from build123d import *

# Parameters (mm, degrees)
SKETCH1_R           = 47.5
BOSS_EXTRUDE1_DEPTH = 100
SKETCH2_R           = 47.5
BOSS_EXTRUDE2_DEPTH = 62.5
SKETCH3_R           = 27
CUT_EXTRUDE1_DEPTH  = 4
HOLE1_D             = 10
HOLE1_DEPTH         = 20
SKETCH6_R           = 30
CUT_EXTRUDE2_DEPTH  = 200


with BuildPart() as part:
    # Sketch1 → Boss-Extrude1 (new body, symmetric)
    with BuildSketch(Plane.XY):
        Circle(SKETCH1_R)
    extrude(amount=BOSS_EXTRUDE1_DEPTH, both=True)

    # Sketch2 → Boss-Extrude2 (add)
    with BuildSketch(Plane(origin=(0, 0, 0), x_dir=(1, 0, 0), z_dir=(0, 1, 0))):
        Circle(SKETCH2_R)
    extrude(amount=BOSS_EXTRUDE2_DEPTH)

    # Sketch3 → Cut-Extrude1 (cut)
    with BuildSketch(Plane(origin=(0, 62.5, 0), x_dir=(1, 0, 0), z_dir=(0, 1, 0))):
        Circle(SKETCH3_R)
    extrude(amount=-CUT_EXTRUDE1_DEPTH, mode=Mode.SUBTRACT)

    # Hole1
    with Locations(Plane(origin=(38, 62.5, 0), x_dir=(0, 0, 1), z_dir=(0, 1, 0))):
        with Locations((0, 0), (-38, -38), (0, -76), (38, -38)):
            Hole(HOLE1_D / 2, depth=HOLE1_DEPTH)

    # Sketch6 → Cut-Extrude2 (cut)
    with BuildSketch(Plane(origin=(0, 0, -100), x_dir=(-1, 0, 0), z_dir=(0, 0, -1))):
        Circle(SKETCH6_R)
    extrude(amount=-CUT_EXTRUDE2_DEPTH, mode=Mode.SUBTRACT)


solid = part.part
Geometry: final body of the model. Coordinates: model frame, mm. A direction names the side the tool comes from. Give positions to 0.01 mm unless a question says otherwise; leave off trailing zeros. Write each loop counter-clockwise with the first axis right and the second up, starting at its lowest first coordinate (ties: lowest second). Pieces come first, ordered by that corner, then holes. Notation, with made-up numbers: (89.5, 56) -> (124.5, 56) arc R32 cw to (124.5, 85) -> close; hole circle Ø3 at (64.5, 35.25). An arc over 180 degrees is marked (long way). Answer as a JSON object with one key per item and string values.
1. Contact query for flat-ended pins moving along their axis: pin 1 (3 mm diameter, centred on x = -0.5, z = -40.5, fed in from +Y); pin 2 (3 mm diameter, centred on x = 23.5, z = 67.5, fed in from +Y); pin 3 (12 mm diameter, centred on x = 24, y = 45.5, fed in from +Z); pin 4 (5 mm diameter, centred on x = -37, z = 11, fed in from -Y). Output: stop coordinate, or through.
Ans:
{"pin 1": "stops at y = 42.5", "pin 2": "stops at y = 42.1", "pin 3": "stops at z = 100", "pin 4": "stops at y = -32.65"}
2. Cut plane B-B on x = 0. Output: boundary loops of the cut face in (y, z), and give its area (3 significant figures).
Ans:
{"outline": "(-47.5, -100) -> (-30, -100) -> (-30, 100) -> (-47.5, 100) -> close; (30, -100) -> (47.5, -100) -> (47.5, -47.5) -> (62.5, -47.5) -> (62.5, -43) -> (42.5, -43) -> (42.5, -33) -> (62.5, -33) -> (62.5, -27) -> (58.5, -27) -> (58.5, 27) -> (62.5, 27) -> (62.5, 33) -> (42.5, 33) -> (42.5, 43) -> (62.5, 43) -> (62.5, 47.5) -> (47.5, 47.5) -> (47.5, 100) -> (30, 100) -> close", "area": "7,810 mm^2"}
3. Cut plane A-A on z = 0. Output: boundary loops of the cut face in (x, y).
Ans:
{"outline": "(-47.5, 0) arc R47.5 ccw to (47.5, 0) -> (47.5, 62.5) -> (43, 62.5) -> (43, 42.5) -> (33, 42.5) -> (33, 62.5) -> (27, 62.5) -> (27, 58.5) -> (-27, 58.5) -> (-27, 62.5) -> (-33, 62.5) -> (-33, 42.5) -> (-43, 42.5) -> (-43, 62.5) -> (-47.5, 62.5) -> close; hole circle Ø60 at (0, 0)"}
4. Cut plane D-D on x = 38. Output: boundary loops of the cut face in (y, z).
Ans:
{"outline": "(-28.5, -100) -> (28.5, -100) -> (28.5, -28.5) -> (62.5, -28.5) -> (62.5, -5) -> (42.5, -5) -> (42.5, 5) -> (62.5, 5) -> (62.5, 28.5) -> (28.5, 28.5) -> (28.5, 100) -> (-28.5, 100) -> close"}
5. Mould query, pull axis Y, two halves, no side actions, for faces 3 (the cylindrical face through (-34, 52, -3)), 4 (the flat face through (-38, 42.5, 0)), 5 (the cylindrical face through (-10.3, -46.37, 1.4)), 6 (the cylindrical face through (29.97, 1.32, -1.4)). Classes: pulls with the +Y half, pulls with the -Y half, needs draft (parallel to the pull), parting line crosses it, or undercut.
Ans:
{"face 3": "needs draft", "face 4": "pulls with the +Y half", "face 5": "parting line crosses it", "face 6": "undercut"}
6. Access query for faces 1 (the flat face through (0, 42.5, -38)), 2 (the flat face through (31, 1, -100)). Directions: +Z, -Z, +X, -X, +Y, -Y. A direction counts if a zero-diameter tool reaches every point of the face in a straight line with its end or side. Return the directions, or none.
Ans:
{"face 1": "+Y", "face 2": "-Z, +X, -X, +Y, -Y"}
7. Ray query, probe 1 along X at (y, z) = (59, 0); probe 2 along X at (y, z) = (51.75, 0); probe 3 along Y at (x, z) = (0, 19.5). Return the intervals inside material, ascending. Write a range as from..to.
Ans:
{"probe 1": "x = -47.5..-43, -33..-27, 27..33, 43..47.5", "probe 2": "x = -47.5..-43, -33..33, 43..47.5", "probe 3": "y = -47.5..-30, 30..58.5"}
8. Cut plane C-C on y = 3. Output: boundary loops of the cut face in (x, z).
Ans:
{"outline": "(-47.41, -100) -> (-29.85, -100) -> (-29.85, 100) -> (-47.41, 100) -> (-47.41, 3) arc R47.5 ccw to (-47.41, -3) -> close; (29.85, -100) -> (47.41, -100) -> (47.41, -3) arc R47.5 ccw to (47.41, 3) -> (47.41, 100) -> (29.85, 100) -> close"}
